Read the model definition and answer for the solid it produces. Units are mm, in the model's axes. Round coordinates to 2 decimals unless told otherwise and drop trailing zeros. Loops run counter-clockwise (first coordinate to the right, second up) from the corner with the lowest first, then second, coordinate; pieces in that order, holes last. Notation, with made-up numbers: (-5, 28.25) - (48, 28.25) arc R32 ccw to (48, 62.25) - close; hole circle Ø8 at (29, 50). An arc over 180 degrees is marked (long way). Answer as CSV lines item,"result".
Autodesk Inventor part; units mm, degrees
ref_plane "YZ Plane" through (0, 0, 0) normal (1, 0, 0) x (0, 1, 0)
ref_plane "XZ Plane" through (0, 0, 0) normal (0, 1, 0) x (-1, 0, 0)
ref_plane "XY Plane" through (0, 0, 0) normal (0, 0, 1) x (1, 0, 0)
sketch "Sketch1" plane through (0, 0, 0) normal (0, 0, 1) x (1, 0, 0)
  line L0 (0, 0) -> (2200, 0)
  line L1 (0, 0) -> (0, -3)
  line L2 (0, -3) -> (2200, -3)
  line L3 (2200, -3) -> (2200, 0)
  dimension "d0" = 2200
  dimension "d1" = 3
  dimension "d2" = 2200
extrude "Extrusion1" add sketch "Sketch1" along normal blind 50
sketch "Sketch2" plane through (0, 0, 0) normal (0, 1, 0) x (1, 0, 0)
  line L0 (0, 0) -> (0, -50)
  line L1 (0, -3) -> (2200, -3)
  line L2 (2200, 0) -> (0, 0)
  line L3 (0, -3) -> (0, 0)
  line L4 (0, 0) -> (2200, 0)
  line L5 (2200, 0) -> (2200, -50)
  line L6 (2200, 0) -> (2200, -3)
  dimension "d5" = 2200
  dimension "d6" = 3
extrude "Extrusion2" add sketch "Sketch2" along normal blind 97
sketch "Sketch3" plane through (0, 0, 3) normal (0, 0, 1) x (1, 0, 0)
  line L0 (0, -3) -> (0, 97)
  line L1 (0, 94) -> (2200, 94)
  line L2 (0, 97) -> (2200, 97)
  line L3 (0, 94) -> (0, 97)
  line L4 (0, 97) -> (2200, 97)
  line L5 (2200, 97) -> (2200, 94)
  point P0 (0, 0)
  dimension "d9" = 3
  dimension "d10" = 2200
extrude "Extrusion3" add sketch "Sketch3" along normal blind 47
fillet "Fillet1" radius 3 4 edges at (1100, -3, 0) (1100, 97, 0) (1100, 0, 3) (1100, 94, 3)
sketch "Sketch4" plane through (0, 0, 0) normal (0, 0, -1) x (-1, 0, 0)
  line L0 (0, 0) -> (0, 94)
  line L1 (-55, 52) -> (-250, 52)
  line L2 (-255.2761, 47.6162) -> (-255.2761, 46.4034)
  line L3 (-250.626, 42.0196) -> (-54.5576, 42.0196)
  arc A0 (-250, 52) -> (-250, 42.0196) centre (-250.313, 47.0098) ccw
  arc A1 (-55.4424, 42.0196) -> (-55, 52) centre (-55, 47) ccw
  dimension "d16" = 10
extrude "Extrusion4" cut sketch "Sketch4" against normal through all contours A1 L3 A0 L2 L1
sketch "Sketch5" plane through (0, 0, 0) normal (0, 0, -1) x (-1, 0, 0)
  line L0 (-2200, 3) -> (-2200, 91)
  line L1 (-2145, 42) -> (-1955, 42)
  line L2 (-1955, 52) -> (-2145, 52)
  arc A0 (-2145, 52) -> (-2145, 42) centre (-2145, 47) ccw
  arc A1 (-1955, 42) -> (-1955, 52) centre (-1955, 47) ccw
  point P0 (0, 0)
extrude "Extrusion5" cut sketch "Sketch5" against normal blind 10
sketch "Sketch8" plane through (0, 0, 0) normal (0, 0, -1) x (-1, 0, 0)
  point P0 (0, 0)
sketch "Sketch9" plane through (0, 0, 0) normal (0, 0, -1) x (-1, 0, 0)
  arc A0 (-1155, 52) -> (-1165, 52) centre (-1160, 52) ccw
  arc A1 (-1116, 52) -> (-1126, 52) centre (-1121, 52) ccw
  arc A2 (-1004, 52) -> (-1014, 52) centre (-1009, 52) ccw
  arc A3 (-965, 52) -> (-975, 52) centre (-970, 52) ccw
  line L0 (-1160, 52) -> (-1160, 47)
  circle A4 centre (-1160, 47) radius 5
  line L1 (-1160, 47) -> (-965, 47)
  line L2 (-1121, 57) -> (-1121, 47)
  line L3 (-1009, 57) -> (-1009, 47)
  line L4 (-970, 57) -> (-970, 47)
  circle A5 centre (-1121, 47) radius 5
  circle A6 centre (-1009, 47) radius 5
  circle A7 centre (-970, 47) radius 5
  point P0 (0, 0)
extrude "Extrusion7" cut sketch "Sketch9" against normal through all
properties part number "ThanhKe"
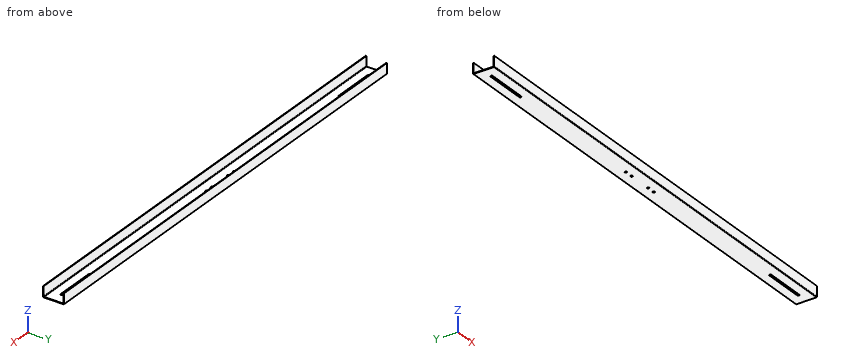
1) A cutting plane is placed at C-C, the plane x = 686.5. Determine the outline of the cut face in (y, z), plus the area to 3 significant figures.
Entries:
outline,"(-3, 3) arc R3 ccw to (0, 0) - (94, 0) arc R3 ccw to (97, 3) - (97, 50) - (94, 50) - (94, 6) arc R3 cw to (91, 3) - (3, 3) arc R3 cw to (0, 6) - (0, 50) - (-3, 50) - close"
area,"582 mm^2"
2) Find the intervals of material crossed by line 1 (Y direction, x = 785.5, z = 18); line 2 (Z direction, x = 251, y = 20); line 3 (Y direction, x = 1160, z = 1), in increasing order.
Entries:
line 1,"y = -3 to 0, 94 to 97"
line 2,"z = 0 to 3"
line 3,"y = -2.24 to 42, 52 to 96.24"
3) A cutting plane is placed at A-A, the plane z = 35. Determine the outline of the cut face in (x, y), plus the area to 3 significant figures.
Entries:
outline,"(0, -3) - (2200, -3) - (2200, 0) - (0, 0) - close; (0, 94) - (2200, 94) - (2200, 97) - (0, 97) - close"
area,"13,200 mm^2"
4) A cutting plane is placed at B-B, the plane x = 164.5. Determine the outline of the cut face in (y, z).
Entries:
outline,"(-3, 3) arc R3 ccw to (0, 0) - (42.02, 0) - (42.02, 3) - (3, 3) arc R3 cw to (0, 6) - (0, 50) - (-3, 50) - close; (52, 0) - (94, 0) arc R3 ccw to (97, 3) - (97, 50) - (94, 50) - (94, 6) arc R3 cw to (91, 3) - (52, 3) - close"
5) A cutting plane is placed at D-D, the plane y = 24.5. Determine the outline of the cut face in (x, z).
Entries:
outline,"(0, 0) - (2200, 0) - (2200, 3) - (0, 3) - close"
6) Each of these flat-tipped pins is pushed along its axis until it touches: P1, Ø16, axis at x = 1121, y = 47, coming from the +Z side; P2, Ø0.9, axis at x = 2013.5, z = 2, coming from the -Y side; P3, Ø3.5, axis at x = 2024, z = 1, coming from the +Y side. Where does it stop, or does it pass through?
Entries:
P1,"stops at z = 3"
P2,"stops at y = -2.95"
P3,"stops at y = 96.99"
